```python
from build123d import *

# Parameters (mm, degrees)
F1_DEPTH = 63.5
F0_W     = 25.4
F0_H     = 19.05
F2_DEPTH = 25.4
F3_DEPTH = 7.9375
F5_R     = 6.35


with BuildPart() as f1:
    # F0 (on Front) → F1 (new body, symmetric)
    with BuildSketch(Plane.XZ):
        Polygon((-41.275, -9.525), (41.275, -9.525), (41.275, 9.525), (22.225, 9.525), (-41.275, 9.525), align=None)
    extrude(amount=F1_DEPTH, both=True)

    # F0 (on Front) → F2 (join, symmetric)
    with BuildSketch(Plane.XZ):
        with BuildLine():
            Line((22.225, 9.525), (41.275, 9.525))
            Line((41.275, 9.525), (41.275, 27.10419))
            ThreePointArc((41.275, 27.10419), (45.92468, 38.32951), (57.15, 42.97919))
            Line((57.15, 42.97919), (60.325, 42.97919))
            Line((60.325, 42.97919), (60.325, 62.02919))
            Line((60.325, 62.02919), (57.15, 62.02919))
            ThreePointArc((57.15, 62.02919), (32.454296, 51.799894), (22.225, 27.10419))
            Line((22.225, 27.10419), (22.225, 9.525))
        make_face()
        with Locations((73.025, 52.50419)):
            Rectangle(F0_W, F0_H)
    extrude(amount=F2_DEPTH, both=True)

    # F0 (on Front) → F3 (join, symmetric)
    with BuildSketch(Plane.XZ):
        with BuildLine():
            add(Edge.make_bspline(
                [(-41.275, 9.525), (-34.716684, 52.690328), (18.733253, 68.238799), (60.325, 62.02919)],
                knots=[0, 0, 0, 0, 114.364549, 114.364549, 114.364549, 114.364549], degree=3))
            Line((-41.275, 9.525), (22.225, 9.525))
            Line((22.225, 9.525), (22.225, 27.10419))
            ThreePointArc((22.225, 27.10419), (32.454296, 51.799894), (57.15, 62.02919))
            Line((57.15, 62.02919), (60.325, 62.02919))
        make_face()
    extrude(amount=F3_DEPTH, both=True)

    # F0 (on Front) → F4 (revolve)
    with BuildSketch(Plane.XZ):
        Polygon((85.725, 66.675), (85.725, 62.02919), (85.725, 42.97919), (85.725, 38.1), (111.125, 38.1), (111.125, 66.675), align=None)
    revolve(axis=Axis((85.725, 0, 52.3875), (0, 0, 1)))

    # F5
    f5_edges = [f1.edges().sort_by_distance(p)[0] for p in [
        (41.275, -63.5, 0),
        (41.275, 63.5, 0),
        (-41.275, -63.5, 0),
        (-41.275, 63.5, 0),
    ]]
    fillet(f5_edges, radius=F5_R)


solid = f1.part
```
The listing builds one solid part. Answer for the finished solid, in the listing's coordinates (mm). A direction names the side the tool comes from. Give positions to 0.01 mm unless a question says otherwise; leave off trailing zeros. Order: outer loops, then holes, each group sorted by start corner. A loop starts at its lowest first (then second) coordinate and runs counter-clockwise, first axis right, second up. Notation, with made-up numbers: (29.25, -29.75) - (38.25, -29.75) arc R27 ccw to (38.25, 9.25) - close; hole circle Ø11 at (-18, -3). An arc over 180 degrees is marked (long way). Answer in a Markdown table with one row per item. Add a question column.
Q1. Find the intervals of material crossed by line 1 along Z through (x, y) = (9, 21.5) (3 decimals); line 2 along Y through (x, z) = (-33, 27); line 3 along X through (y, z) = (-5.5, 5) (3 decimals), in increasing order. Write a range as [from, to].
Q2. The part is cut by section B-B (x = 67). Determine the outline of the cut face in (y, z) (3 decimals).
Q3. The part is cut by section C-C (y = 49). Determine the outline of the cut face in (x, z) (3 decimals).
Q4. The part is cut by section A-A (y = -17). Determine the outline of the cut face in (x, z) (3 decimals).
Q5. Which of the six approach directions +Z, -Z, +X, -X, +Y, -Y give full straight-line access (tool end or side, diameter ignored) to faces 1 (the flat face through (46, -25.4, 42)), 2 (the flat face through (22.225, 17, 18)), 3 (the flat face through (46, 25.4, 42)), 4 (the cylindrical face through (32.73, -16.79, 52.07))?
Q6. The part is cut by section D-D (x = 101.5). Determine the outline of the cut face in (y, z) (3 decimals), then the cut area to 3 significant figures.
Q7. Given P1, Ø1.5, axis at x = 82.5, y = -4.5, coming from the -Z side; P2, Ø1, axis at x = -19.5, z = 34.5, coming from the -Y side; P3, Ø1, axis at x = 19.5, y = 6, coming from the +Z side, each flat-ended and moving along its own axis, determine where each tip first touches the part or whether it passes through.
Q8. For a pull along X with two mould halves and no side action, classify faces 5 (the flat face through (60, 2, 42.979)), 6 (the cylindrical face through (-39.365, -61.689, -0.133)), 7 (the cylindrical face through (39.464, -61.59, 0.133)) as released by +X, released by -X, zero draft, split by the parting line, or undercut.
Determined:
| question | item | result |
|---|---|---|
| 1 | line 1 | z = [-9.525, 9.525] |
| 1 | line 2 | y = [-7.94, 7.94] |
| 1 | line 3 | x = [-41.275, 41.275] |
| 2 | outline | (-25.4, 42.979) - (-17.162, 42.979) - (-17.162, 38.1) - (17.162, 38.1) - (17.162, 42.979) - (25.4, 42.979) - (25.4, 62.029) - (17.162, 62.029) - (17.162, 66.675) - (-17.162, 66.675) - (-17.162, 62.029) - (-25.4, 62.029) - close |
| 3 | outline | (-41.275, -9.525) - (41.275, -9.525) - (41.275, 9.525) - (-41.275, 9.525) - close |
| 4 | outline | (-41.275, -9.525) - (41.275, -9.525) - (41.275, 27.104) arc R15.875 cw to (57.15, 42.979) - (66.853, 42.979) - (66.853, 38.1) - (104.597, 38.1) - (104.597, 66.675) - (66.853, 66.675) - (66.853, 62.029) - (57.15, 62.029) arc R34.925 ccw to (22.225, 27.104) - (22.225, 9.525) - (-41.275, 9.525) - close |
| 5 | face 1 | +Z, +X, -X, -Y |
| 5 | face 2 | +Z, -X, +Y |
| 5 | face 3 | +Z, +X, -X, +Y |
| 5 | face 4 | +Z, -X, -Y |
| 6 | outline | (-19.908, 38.1) - (19.908, 38.1) - (19.908, 66.675) - (-19.908, 66.675) - close |
| 6 | area | 1,140 mm² |
| 7 | P1 | stops at z = 38.1 |
| 7 | P2 | stops at y = -7.94 |
| 7 | P3 | stops at z = 61.36 |
| 8 | face 5 | undercut |
| 8 | face 6 | released by -X |
| 8 | face 7 | released by +X |
